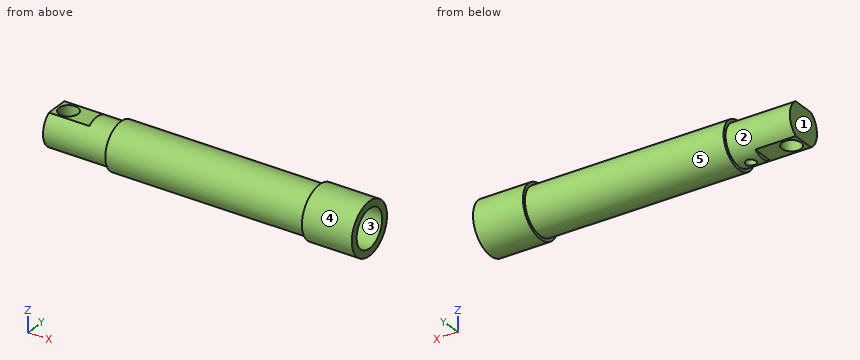
```python
from build123d import *

# Parameters (mm, degrees)
SKETCH2_R           = 26.9875
BOSS_EXTRUDE1_DEPTH = 85.725
CUT_EXTRUDE1_DEPTH  = 53.975
SKETCH4_R           = 12.7
CUT_EXTRUDE2_DEPTH  = 58.15
SKETCH8_R           = 12.7
CUT_EXTRUDE3_DEPTH  = 26.9875


with BuildPart() as part:
    # Sketch1 → Revolve1 (revolve)
    with BuildSketch(Plane.XY):
        Polygon((165.89375, 34.925), (99.21875, 34.925), (99.21875, 30.95625), (-165.89375, 30.95625), (-165.89375, 25.4), (165.89375, 25.4), align=None)
    revolve(axis=Axis((-165.89375, 0, 0), (1, 0, 0)))

    # Sketch2 → Boss-Extrude1 (add)
    with BuildSketch(Plane.ZY.offset(165.89375)):
        Circle(SKETCH2_R)
    extrude(amount=BOSS_EXTRUDE1_DEPTH)

    # Sketch3 → Cut-Extrude1 (cut)
    with BuildSketch(Plane.ZY.offset(251.61875)):
        with BuildLine():
            Line((-22.225, 15.309295583), (-22.225, -15.309295583))
            ThreePointArc((-22.225, -15.309295583), (-26.9875, 0), (-22.225, 15.309295583))
        make_face()
        with BuildLine():
            Line((22.225, 15.309295583), (22.225, -15.309295583))
            ThreePointArc((22.225, -15.309295583), (26.9875, 0), (22.225, 15.309295583))
        make_face()
    extrude(amount=-CUT_EXTRUDE1_DEPTH, mode=Mode.SUBTRACT)

    # Sketch4 → Cut-Extrude2 (cut, through all)
    with BuildSketch(Plane.XY.offset(22.225)):
        with Locations((-235.74375, 0)):
            Circle(SKETCH4_R)
    extrude(amount=-CUT_EXTRUDE2_DEPTH, mode=Mode.SUBTRACT)

    # Sketch6 → 1/4 NPT Tapped Hole1 (revolve, cut)
    with BuildSketch(Plane(origin=(-181.76875, 0, -26.9875), x_dir=(0, 1, 0), z_dir=(1, 0, 0))):
        Polygon((0, 0), (0, 20.411147279), (5.5626, 17.0688), (5.5626, 10.0203), (6.557978799, 10.0203), (6.858, 0), align=None)
    revolve(axis=Axis((-181.76875, 0, -33.3375), (0, 0, 1)), mode=Mode.SUBTRACT)

    # Sketch8 → Cut-Extrude3 (cut)
    with BuildSketch(Plane(origin=(-165.89375, 0, 0), x_dir=(0, 0, -1), z_dir=(1, 0, 0))):
        Circle(SKETCH8_R)
    extrude(amount=-CUT_EXTRUDE3_DEPTH, mode=Mode.SUBTRACT)


solid = part.part
```
Can you work these out from the model? Positions are in its coordinate system, mm. Face numbers are marked on the shaded views. A direction names the side the tool comes from. Coordinates: 2 decimals unless noted, no trailing zeros. Order: outer loops, then holes, each group sorted by start corner. A loop starts at its lowest first (then second) coordinate and runs counter-clockwise, first axis right, second up.
1. If we section it at D-D (x = -54.5): Please give me the cut outline in (y, z).
2. If we section it at B-B (x = 130): Please give me the cut outline in (y, z) (3 decimals).
3. I'm going to push flat-ended pins straight in: pin 1 (12 mm diameter, centred on x = -42, y = -23, fed in from +Z); pin 2 (1.5 mm diameter, centred on y = 18.5, z = 6, fed in from +X); pin 3 (1.4 mm diameter, centred on y = 3, z = 25.5, fed in from -X). Where does each tip first touch, or does it pass through?
4. Thinking about a two-plate mould opening in Y: for the marked faces 1, 2 and 3, which applies, +Y half, -Y half, draft (parallel to the pull), parting line (faces both ways), or undercut?
5. I need wall thicknesses on line 1 (Z direction, x = -159, y = 0.5); line 2 (Z direction, x = 114, y = 0) (3 decimals); line 3 (X direction, y = 16, z = 0.5). Which ranges of each line are inside material? Lowest first, please.
6. If we section it at A-A (z = 0): Please give me the cut outline in (x, y) (1 decimal).
7. For the marked faces 4 and 5, which set-ups out of +Z, -Z, +X, -X, +Y, -Y let a thin tool reach every point of the face, with its end or its side?
8. If we section it at C-C (y = 0): Give the number of separate pieces and of enclosed holes in the cut face, then the cut area to 3 significant figures.
Entries:
1. outline: circle Ø61.91 at (0, 0); hole circle Ø50.8 at (0, 0)
2. outline: circle Ø69.85 at (0, 0); hole circle Ø50.8 at (0, 0)
3. pin 1: stops at z = 25.87
3. pin 2: stops at x = -165.89
3. pin 3: stops at x = -197.64
4. face 1: draft
4. face 2: parting line
4. face 3: undercut
5. line 1: z = -30.95 to -25.4, 25.4 to 30.95
5. line 2: z = -34.925 to -25.4, 25.4 to 34.925
5. line 3: x = -251.62 to -165.89
6. outline: (-251.6, -27) - (-165.9, -27) - (-165.9, -31) - (99.2, -31) - (99.2, -34.9) - (165.9, -34.9) - (165.9, -25.4) - (-165.9, -25.4) - (-165.9, -12.7) - (-192.9, -12.7) - (-192.9, 12.7) - (-165.9, 12.7) - (-165.9, 25.4) - (165.9, 25.4) - (165.9, 34.9) - (99.2, 34.9) - (99.2, 31) - (-165.9, 31) - (-165.9, 27) - (-251.6, 27) - close; hole circle Ø25.4 at (-235.7, 0)
7. face 4: +X, -X
7. face 5: -X
8. separate pieces: 3
8. enclosed holes: 0
8. area: 6,330 mm2
